Geometry: final body of the model. Coordinates: model frame, mm. A direction names the side the tool comes from. Give positions to 0.01 mm unless a question says otherwise; leave off trailing zeros. Order: outer loops, then holes, each group sorted by start corner. A loop starts at its lowest first (then second) coordinate and runs counter-clockwise, first axis right, second up. Notation, with made-up numbers: M -12.75,7.25 L 32.25,7.25 A29 ccw 32.25,41.25 Z; hole C 0,23 d11. An arc over 180 degrees is marked long. One line per item, written item: value. Start each with the question number.
```python
from build123d import *

# Parameters (mm, degrees)
BOSS_EXTRUDE1_DEPTH = 0.285
SKETCH2_W           = 4.9
SKETCH2_H           = 6.35
BOSS_EXTRUDE2_DEPTH = 2
BOSS_EXTRUDE3_DEPTH = 1.555
SKETCH4_W           = 0.635
SKETCH4_H           = 0.635
BOSS_EXTRUDE4_DEPTH = 8.85


with BuildPart() as part:
    # Sketch1 → Boss-Extrude1 (new, symmetric)
    with BuildSketch(Plane(origin=(0, 0, 0), x_dir=(1, 0, 0), z_dir=(0, 1, 0))):
        with BuildLine():
            Line((8.256488358, 3.85), (46.598758561, 3.85))
            Line((46.598758561, 3.85), (47.998758561, 2.45))
            Line((47.998758561, 2.45), (52.06, 2.45))
            Line((52.06, 2.45), (52.06, -2.45))
            Line((52.06, -2.45), (47.998758561, -2.45))
            Line((47.998758561, -2.45), (46.598758561, -3.85))
            Line((46.598758561, -3.85), (8.256488358, -3.85))
            ThreePointArc((8.256488358, -3.85), (-9.11, 0), (8.256488358, 3.85))
        make_face()
    extrude(amount=BOSS_EXTRUDE1_DEPTH, both=True)

    # Sketch2 → Boss-Extrude2 (add)
    with BuildSketch(Plane(origin=(52.06, 0, 0), x_dir=(0, 0, -1), z_dir=(1, 0, 0))):
        Rectangle(SKETCH2_W, SKETCH2_H)
    extrude(amount=BOSS_EXTRUDE2_DEPTH)

    # Sketch3 → Boss-Extrude3 (add, symmetric)
    with BuildSketch(Plane.XY):
        Polygon((54.06, 3.175), (60.27, 3.175), (60.27, 2.355), (58.79, 1.405), (57.54, 1.405), (56.06, 2.355), (54.06, 2.355), align=None)
    extrude(amount=BOSS_EXTRUDE3_DEPTH, both=True)

    # Sketch4 → Boss-Extrude4 (add)
    with BuildSketch(Plane(origin=(54.06, 0, 0), x_dir=(0, 0, -1), z_dir=(1, 0, 0))):
        with Locations((-1.27, 0)):
            Rectangle(SKETCH4_W, SKETCH4_H)
        with Locations((1.27, 0)):
            Rectangle(SKETCH4_W, SKETCH4_H)
    extrude(amount=BOSS_EXTRUDE4_DEPTH)


solid = part.part
```
Q1. Section query B-B on x = 0. Return loops of the section in (y, z) (3 decimals).
Q2. Mould query, pull axis X, two halves, no side actions, for faces 4 (the face through (54.06, 0, 0)), 5 (the face through (59.54, 1.887, 0.022)), 6 (the face through (57, 2, -1.555)). Classes: +X half, -X half, draft (parallel to the pull), parting line (faces both ways), or undercut.
Q3. Ray query, line 1 along X through (y, z) = (-1.5, -2.25); line 2 along Y through (x, z) = (36, -3) (3 decimals); line 3 along Z through (x, y) = (50, -0.25). Return the intervals inside material, ascending. Write a range as [from, to].
Q4. Section query A-A on z = 0. Return loops of the section in (x, y) (3 decimals), and give its area (3 significant figures).
Q5. Set-up query: faces 1 (the face through (58, 1.405, 0)), 2 (the face through (56.81, 1.873, 0.022)), 3 (the face through (15, -0.285, 0)). Return all of +Z, -Z, +X, -X, +Y, -Y with unobstructed straight access to the full face (end or side cutting, diameter ignored); none if empty.
Q6. Contact query for flat-ended pins moving along their axis: pin 1 (1.5 mm diameter, centred on y = -0.5, z = 2.5, fed in from +X); pin 2 (2 mm diameter, centred on y = 1, z = 1.5, fed in from -X); pin 3 (2 mm diameter, centred on y = -1, z = -6.5, fed in from +X); pin 4 (0.7 mm diameter, centred on x = 60.5, z = -1.5, fed in from +Y) (3 decimals). Output: stop coordinate, or through.
Q7. Section query C-C on x = 17.5. Return loops of the section in (y, z) (3 decimals).
Results below:
1. outline: M -0.285,-9.11 L 0.285,-9.11 L 0.285,9.11 L -0.285,9.11 Z
2. face 4: undercut
2. face 5: +X half
2. face 6: draft
3. line 1: [52.06, 54.06]
3. line 2: [-0.285, 0.285]
3. line 3: [-2.45, 2.45]
4. outline: M -9.11,-0.285 L 52.06,-0.285 L 52.06,-3.175 L 54.06,-3.175 L 54.06,2.355 L 56.06,2.355 L 57.54,1.405 L 58.79,1.405 L 60.27,2.355 L 60.27,3.175 L 52.06,3.175 L 52.06,0.285 L -9.11,0.285 Z
4. area: 55.3 mm2
5. face 1: +Z, -Z, +X
5. face 2: +Z, -Z
5. face 3: +Z, -Z, -X, -Y
6. pin 1: x = 54.06
6. pin 2: x = -9.07
6. pin 3: x = 7.02
6. pin 4: y = 3.175
7. outline: M -0.285,-3.85 L 0.285,-3.85 L 0.285,3.85 L -0.285,3.85 Z
